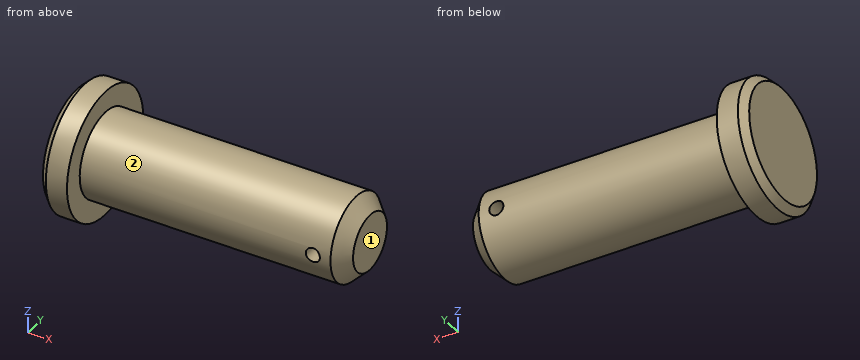
from build123d import *

# Parameters (mm, degrees)
F2_SIZE  = 4
F3_SIZE  = 2
F4_R     = 2
F5_DEPTH = 12.5


with BuildPart() as f1:
    # F0 (on Front) → F1 (revolve)
    with BuildSketch(Plane.XZ):
        Polygon((75, 12), (0, 12), (0, 18), (-8, 18), (-8, 0), (75, 0), align=None)
    revolve(axis=Axis((33.5, 0, 0), (1, 0, 0)))

    # F2
    f2_edges = [f1.edges().sort_by_distance(p)[0] for p in [
        (75, 0, -12),
    ]]
    chamfer(f2_edges, length=F2_SIZE)

    # F3
    f3_edges = [f1.edges().sort_by_distance(p)[0] for p in [
        (-8, 0, -18),
    ]]
    chamfer(f3_edges, length=F3_SIZE)

    # F4 (on Front) → F5 (cut, symmetric)
    with BuildSketch(Plane.XZ):
        with Locations((66, 0)):
            Circle(F4_R)
    extrude(amount=F5_DEPTH, both=True, mode=Mode.SUBTRACT)


solid = f1.part
Source: CAD feature listing. Evaluate the final solid. Frame: model axes, mm. Face numbers are marked on the shaded views. A direction names the side the tool comes from. Give positions to 0.01 mm unless a question says otherwise; leave off trailing zeros. Order: outer loops, then holes, each group sorted by start corner. A loop starts at its lowest first (then second) coordinate and runs counter-clockwise, first axis right, second up. Notation, with made-up numbers: (-25.5, 64) -> (16.5, 64) arc R17 ccw to (16.5, 76) -> close; hole circle Ø4 at (-32, 44). An arc over 180 degrees is marked (long way). Use a Markdown table: item, result.
1) Reachability of the marked faces 1 and 2 from +Z, -Z, +X, -X, +Y, -Y: full face, straight path, thin tool, end or side. Return the list, or none.
Answer list:
| item | result |
|---|---|
| face 1 | +Z, -Z, +X, +Y, -Y |
| face 2 | +X |
2) Section query B-B, the plane y = 0. Return the cut outline in (x, z), then the cut area to 3 significant figures.
Answer list:
| item | result |
|---|---|
| outline | (-8, -16) -> (-6, -18) -> (0, -18) -> (0, -12) -> (71, -12) -> (75, -8) -> (75, 8) -> (71, 12) -> (0, 12) -> (0, 18) -> (-6, 18) -> (-8, 16) -> close; hole circle Ø4 at (66, 0) |
| area | 2,060 mm² |
3) Section query A-A, the plane z = 0. Return the cut outline in (x, y).
Answer list:
| item | result |
|---|---|
| outline | (-8, -16) -> (-6, -18) -> (0, -18) -> (0, -12) -> (64, -12) -> (64, 12) -> (0, 12) -> (0, 18) -> (-6, 18) -> (-8, 16) -> close; (68, -12) -> (71, -12) -> (75, -8) -> (75, 8) -> (71, 12) -> (68, 12) -> close |
4) Section query C-C, the plane x = 62. Return the cut outline in (y, z), then the cut area to 3 significant figures.
Answer list:
| item | result |
|---|---|
| outline | circle Ø24 at (0, 0) |
| area | 452 mm² |
5) Contact query for flat-ended pins moving along their axis: P1, Ø10, axis at x = 62.5, z = 11.5, coming from the -Y side; P2, Ø12, axis at x = 59.5, y = -7.5, coming from the -Z side; P3, Ø3, axis at x = 62.5, y = 1.5, coming from the -Z side. Output: stop coordinate, or through.
Answer list:
| item | result |
|---|---|
| P1 | y = -10.09 |
| P2 | z = -11.91 |
| P3 | z = -12 |
6) Ray query, line 1 along X through (y, z) = (-2.5, 0); line 2 along Z through (x, y) = (66, -1); line 3 along Z through (x, y) = (66, -6.75). Return the intervals inside material, ascending. Write a range as [from, to].
Answer list:
| item | result |
|---|---|
| line 1 | [-8, 64], [68, 75] |
| line 2 | [-11.96, -2], [2, 11.96] |
| line 3 | [-9.92, -2], [2, 9.92] |
